Could you check a few things on this model? Use its own coordinates, in mm. A direction names the side the tool comes from. Round coordinates to 2 decimals unless told otherwise and drop trailing zeros. Loops run counter-clockwise (first coordinate to the right, second up) from the corner with the lowest first, then second, coordinate; pieces in that order, holes last. Notation, with made-up numbers: (54.5, 18.25) -> (102.5, 18.25) arc R19 cw to (102.5, 35.25) -> close; hole circle Ø2 at (-10.75, -4). An arc over 180 degrees is marked (long way). One line per item, written item: value.
Autodesk Inventor part; units mm, degrees
ref_plane "РабПлоскость1" through (3.555, 0, 1.4115) normal (1, 0, 0) x (0, 1, 0)
ref_plane "РабПлоскость10" through (3.555, 0, 1.4115) normal (0, 1, 0) x (-1, 0, 0)
ref_plane "РабПлоскость13" through (0, -3.11, 1.4115) normal (-1, 0, 0) x (0, -1, 0)
sketch "Эскиз1" plane through (0, 0, 0) normal (0, 0, 1) x (1, 0, 0)
  line L0 (-3.555, 3.11) -> (3.555, 3.11)
  line L1 (3.555, 3.11) -> (3.555, -3.11)
  line L2 (3.555, -3.11) -> (-3.555, -3.11)
  line L3 (-3.555, -3.11) -> (-3.555, 3.11)
  point P0 (0, 0)
  dimension "d0" = 3.555
  dimension "d1" = 3.11
  dimension "d2" = 7.11
  dimension "d3" = 6.22
extrude "Выдавливание1" add sketch "Эскиз1" along normal blind 2.62
sketch "Эскиз4" plane through (-3.555, -3.11, 0) normal (0, -1, 0) x (1, 0, 0)
  line L0 (7.11, 2.62) -> (0, 2.62)
  line L1 (0, 0) -> (0, 2.62)
  line L2 (7.11, 0) -> (0, 0)
  line L3 (7.11, 0) -> (7.11, 2.62)
  line L4 (0.1057, 2.62) -> (0, 1.4115)
  line L5 (0, 1.4115) -> (0.088, 0.406)
  line L6 (7.0043, 2.62) -> (7.11, 1.4115)
  line L7 (7.11, 1.4115) -> (7.022, 0.406)
  line L8 (0.088, 0.406) -> (1.6, 0.406)
  line L9 (1.6, 0.406) -> (1.6, 0.203)
  line L10 (1.6, 0.203) -> (5.51, 0.203)
  line L11 (5.51, 0.203) -> (5.51, 0.406)
  line L12 (5.51, 0.406) -> (7.022, 0.406)
  point P0 (3.555, 0)
  dimension "d24" = 0.203
  dimension "d25" = 0.203
  dimension "d26" = 1.6
  dimension "d27" = 1.6
  dimension "d28" = 1.2085
  dimension "d29" = 1.2085
  dimension "d30" = 1.2085
  dimension "d31" = 1.2085
  dimension "d32" = 5
  dimension "d33" = 5
  dimension "d34" = 5
  dimension "d35" = 5
extrude "Выдавливание3" cut sketch "Эскиз4" against normal through all contours L3 L6 L0 | L3 L2 L1 L5 L8 L9 L10 L11 L12 L7 | L4 L1 L0
ref_plane "РабПлоскость1" through (3.555, 0, 1.4115) normal (1, 0, 0) x (0, 1, 0)
sketch "Эскиз5" plane through (3.555, 0, 1.4115) normal (1, 0, 0) x (0, 1, 0)
  line L0 (3.11, 1.2085) -> (3.11, 0)
  line L1 (-3.11, 1.2085) -> (3.11, 1.2085)
  line L2 (-3.11, 0) -> (-3.11, 1.2085)
  line L3 (-3.11, 0) -> (3.11, 0)
  line L4 (3.11, 0) -> (3.11, -1.0055)
  line L5 (-3.11, 0) -> (3.11, 0)
  line L6 (-3.11, -1.0055) -> (-3.11, 0)
  line L7 (-3.11, -1.0055) -> (3.11, -1.0055)
  line L8 (-3.11, 0) -> (-3.0043, 1.2085)
  line L9 (3.11, 0) -> (3.0043, 1.2085)
  line L10 (-3.0043, 1.2085) -> (-3.11, 1.2085)
  line L11 (-3.11, 1.2085) -> (-3.11, 0)
  line L12 (3.11, 0) -> (3.11, 1.2085)
  line L13 (3.11, 1.2085) -> (3.0043, 1.2085)
  line L14 (3.11, -1.0055) -> (3.11, -1.2085)
  line L15 (-3.11, -1.0055) -> (3.11, -1.0055)
  line L16 (-3.11, -1.2085) -> (-3.11, -1.0055)
  line L17 (-3.11, -1.2085) -> (3.11, -1.2085)
  line L18 (-3.11, 0) -> (-3.0043, -1.2085)
  line L19 (-3.0043, -1.2085) -> (-3.11, -1.2085)
  line L20 (-3.11, -1.2085) -> (-3.11, 0)
  line L21 (3.11, 0) -> (3.0043, -1.2085)
  line L22 (3.0043, -1.2085) -> (3.11, -1.2085)
  line L23 (3.11, -1.2085) -> (3.11, 0)
  point P0 (0, -1.4115)
  dimension "d39" = 5
  dimension "d40" = 5
  dimension "d43" = 5
  dimension "d44" = 5
extrude "Выдавливание4" cut sketch "Эскиз5" against normal through all contours L0 L9 L1 | L4 L7 L21 | L18 L7 L6 | L2 L1 L8 | L14 L17 L21 L7 | L7 L18 L17 L16
ref_plane "РабПлоскость10" through (3.555, 0, 1.4115) normal (0, 1, 0) x (-1, 0, 0)
ref_plane "РабПлоскость8" through (3.555, -3.11, 1.4115) normal (0, 1, 0) x (-1, 0, 0)
ref_plane "РабПлоскость9" through (0, 3.11, 1.4115) normal (0, 1, 0) x (-1, 0, 0)
sketch "Эскиз7" plane through (3.555, 0, 1.4115) normal (0, 1, 0) x (-1, 0, 0)
  line L0 (0.1057, 1.2085) -> (0, 0)
  line L1 (7.0043, 1.2085) -> (0.1057, 1.2085)
  line L2 (7.11, 0) -> (7.0043, 1.2085)
  line L3 (0, 0) -> (7.11, 0)
  line L4 (0, 0) -> (0.088, -1.0055)
  line L5 (0, 0) -> (7.11, 0)
  line L6 (7.022, -1.0055) -> (7.11, 0)
  line L7 (5.51, -1.0055) -> (7.022, -1.0055)
  line L8 (5.51, -1.2085) -> (5.51, -1.0055)
  line L9 (1.6, -1.2085) -> (5.51, -1.2085)
  line L10 (1.6, -1.0055) -> (1.6, -1.2085)
  line L11 (0.088, -1.0055) -> (1.6, -1.0055)
  line L12 (3.555, -1.4115) -> (3.555, 2.1644) construction
  line L13 (-0.51, -0.3) -> (-0.51, -1.1115)
  line L14 (1.01, -1.4115) -> (-0.21, -1.4115)
  line L15 (1.01, -1.2115) -> (1.01, -1.4115)
  line L16 (1.01, -1.2115) -> (-0.21, -1.2115)
  line L17 (0, 0) -> (-0.21, 0)
  line L18 (0, 0) -> (0.0175, -0.2)
  line L19 (0.0175, -0.2) -> (-0.21, -0.2)
  line L20 (-0.31, -0.3) -> (-0.31, -1.1115)
  arc A0 (-0.31, -1.1115) -> (-0.21, -1.2115) centre (-0.21, -1.1115) ccw
  arc A1 (-0.21, -0.2) -> (-0.31, -0.3) centre (-0.21, -0.3) ccw
  arc A2 (-0.51, -1.1115) -> (-0.21, -1.4115) centre (-0.21, -1.1115) ccw
  arc A3 (-0.21, 0) -> (-0.51, -0.3) centre (-0.21, -0.3) ccw
  line L21 (3.555, -1.4115) -> (1.6, -1.4115) construction
  dimension "d62" = 4.065
  dimension "d64" = 1.52
  dimension "d65" = 0.2
  dimension "d66" = 0.2
  dimension "d67" = 0.2
  dimension "d68" = 0.2
  dimension "d69" = 0.2
extrude "Выдавливание6" add sketch "Эскиз7" along normal mid plane 3.2 contours L4 L19 A1 L20 A0 L16 L15 L14 A2 L13 A3 L17
ref_plane "РабПлоскость13" through (0, -3.11, 1.4115) normal (-1, 0, 0) x (0, -1, 0)
ref_plane "РабПлоскость11" through (3.555, 0, 1.4115) normal (1, 0, 0) x (0, 1, 0)
ref_plane "РабПлоскость12" through (-3.555, -3.11, 1.4115) normal (-1, 0, 0) x (0, -1, 0)
mirror "Зеркальное отражение2" about plane through (0, -3.11, 1.4115) normal (-1, 0, 0) of "Выдавливание6"
equation "\"d25\" = d24"
equation "\"d27\" = d26"
equation "\"d28\" = d29"
equation "\"d30\" = d31"
properties part number "DO-214AB (SMC)"
Item 1: For faces 4 (the face through (3.865, 0, 0.7)), 5 (the face through (3.5, -0.04, 2.02)), 6 (the face through (0, 0, 0.203)), which set-ups out of +Z, -Z, +X, -X, +Y, -Y let a thin tool reach every point of the face, with its end or its side?
Output:
face 4: +Y, -Y
face 5: +Z, +X, +Y, -Y
face 6: -Z, +Y, -Y
Item 2: If we mould it in two halves opening along X, with no side actions, what happens to faces 1 (the face through (0.05, 3.06, 0.82)), 2 (the face through (-4.065, 0, 0.7)), 3 (the face through (3, 0, 0.2))? For each: released by +X, released by -X, zero draft, split by the parting line, or undercut.
Output:
face 1: zero draft
face 2: released by -X
face 3: undercut
Item 3: I need wall thicknesses on line 1 (X direction, y = 0.25, z = 0.95) (3 decimals); line 2 (Z direction, x = 3, y = -0.75); line 3 (Z direction, x = -1.5, y = 0). Which ranges of each line are inside material? Lowest first, please. Write a range as from..to.
Output:
line 1: x = -4.065..-3.865, -3.515..3.515, 3.865..4.065
line 2: z = 0..0.2, 0.41..2.62
line 3: z = 0.2..2.62
Item 4: If we section it at A-A on x = -2.75: List the corners of the cut face in (y, z) for me.
Output:
outline: (-3.11, 1.41) -> (-3.02, 0.41) -> (3.02, 0.41) -> (3.11, 1.41) -> (3, 2.62) -> (-3, 2.62) -> close; (-1.6, 0) -> (1.6, 0) -> (1.6, 0.2) -> (-1.6, 0.2) -> close
Item 5: If we section it at D-D on x = -0.5: List the corners of the cut face in (y, z) for me, plus the area to 3 significant figures.
Output:
outline: (-3.11, 1.41) -> (-3, 0.2) -> (3, 0.2) -> (3.11, 1.41) -> (3, 2.62) -> (-3, 2.62) -> close
area: 14.8 mm²
Item 6: Will these pins go through, and if not, where does the flat tip stop? pin 1 Ø1.2 at (x, y) = (0.5, 1) entering from -Z; pin 2 Ø0.7 at (x, z) = (3.5, 0.5) entering from +Y.
Output:
pin 1: stops at z = 0.2
pin 2: stops at y = 3.06
Item 7: If we section it at B-B on z = 0.85: List the corners of the cut face in (x, y) for me (3 decimals), plus the area to 3 significant figures.
Output:
outline: (-4.065, -1.6) -> (-3.865, -1.6) -> (-3.865, 1.6) -> (-4.065, 1.6) -> close; (-3.506, -3.061) -> (3.506, -3.061) -> (3.506, 3.061) -> (-3.506, 3.061) -> close; (3.865, -1.6) -> (4.065, -1.6) -> (4.065, 1.6) -> (3.865, 1.6) -> close
area: 44.2 mm²
